Autodesk Inventor part; units mm, degrees
ref_plane "YZ Plane" through (0, 0, 0) normal (1, 0, 0) x (0, 1, 0)
ref_plane "XZ Plane" through (0, 0, 0) normal (0, 1, 0) x (-1, 0, 0)
ref_plane "XY Plane" through (0, 0, 0) normal (0, 0, 1) x (1, 0, 0)
sketch "Sketch1" plane through (0, 0, 0) normal (0, 0, 1) x (1, 0, 0)
  line L0 (0, 0) -> (235, 0)
  line L1 (235, 0) -> (235, 51)
  line L2 (235, 51) -> (0, 51)
  line L3 (0, 51) -> (0, 0)
  dimension "d0" = 235
  dimension "d1" = 51
extrude "Extrusion1" add sketch "Sketch1" along normal blind 5
sketch "Sketch2" plane through (0, 0, 5) normal (0, 0, 1) x (1, 0, 0)
  line L0 (0, 0) -> (235, 0)
  line L1 (235, 0) -> (235, 51)
  line L2 (235, 51) -> (0, 51)
  line L3 (0, 51) -> (0, 0)
  line L4 (235, 0) -> (235, 51)
  line L5 (0, 22.5) -> (235, 22.5)
  line L6 (235, 22.5) -> (235, 28.5)
  line L7 (235, 28.5) -> (0, 28.5)
  line L8 (0, 28.5) -> (0, 22.5)
  line L9 (0, 22.5) -> (235, 28.5) construction
  line L10 (235, 22.5) -> (0, 28.5) construction
  point P0 (117.5, 25.5)
  dimension "d4" = 6
extrude "Extrusion2" add sketch "Sketch2" along normal blind 3 contours L3 L7 L1 L5
sketch "Sketch3" plane through (0, 0, 5) normal (0, 0, 1) x (1, 0, 0)
  line L0 (0, 28.5) -> (235, 28.5)
  line L1 (235, 51) -> (0, 51)
  line L2 (34.5, 28.5) -> (39.5, 28.5)
  line L3 (39.5, 28.5) -> (39.5, 51)
  line L4 (39.5, 51) -> (34.5, 51)
  line L5 (34.5, 51) -> (34.5, 28.5)
  point P0 (0, 0)
  dimension "d7" = 5
sketch "Sketch5" plane through (0, 0, 5) normal (0, 0, 1) x (1, 0, 0)
  line L0 (235, 51) -> (0, 51)
  line L1 (117.5, 51) -> (117.5, 0)
  line L2 (235, 28.5) -> (0, 28.5)
  line L3 (34.5, 51) -> (39.5, 51)
  line L4 (39.5, 51) -> (39.5, 28.5)
  line L5 (39.5, 28.5) -> (34.5, 28.5)
  line L6 (34.5, 28.5) -> (34.5, 51)
  line L7 (0, 22.5) -> (235, 22.5)
  line L8 (34.5, 22.5) -> (39.5, 22.5)
  line L9 (39.5, 22.5) -> (39.5, 0)
  line L10 (39.5, 0) -> (34.5, 0)
  line L11 (34.5, 0) -> (34.5, 22.5)
  line L12 (195.5, 51) -> (195.5, 28.5)
  line L13 (200.5, 28.5) -> (200.5, 51)
  line L14 (195.5, 22.5) -> (195.5, 0)
  line L15 (195.5, 0) -> (200.5, 0)
  line L16 (200.5, 0) -> (200.5, 22.5)
  line L17 (195.5, 28.5) -> (200.5, 28.5)
  line L18 (195.5, 22.5) -> (200.5, 22.5)
  line L19 (195.5, 51) -> (200.5, 51)
  point P0 (0, 0)
  dimension "d13" = 5
extrude "Extrusion5" add sketch "Sketch3" along normal blind 3
extrude "Extrusion6" add sketch "Sketch5" along normal blind 3 contours L9 L10 L11 L7
extrude "Extrusion7" add sketch "Sketch5" along normal blind 3 contours L13 L2 L12 L0 | L7 L16 L15 L14
sketch "Sketch8" plane through (0, 0, 5) normal (0, 0, 1) x (1, 0, 0)
  circle A0 centre (29.5, 5.625) radius 1.6
  circle A1 centre (19.5, 16.875) radius 1.6
  line L0 (39.5, 0) -> (39.5, 22.5)
  line L1 (34.5, 22.5) -> (34.5, 0)
  line L2 (0, 0) -> (34.5, 0)
  dimension "d24" = 3.2
  dimension "d25" = 3.2
  dimension "d27" = 5
  dimension "d28" = 5.625
  dimension "d29" = 15
  dimension "d30" = 16.875
extrude "Extrusion9" cut sketch "Sketch8" against normal blind 10
sketch "Sketch9" plane through (0, 0, 8) normal (0, 0, 1) x (1, 0, 0)
  line L0 (0, 51) -> (0, 0)
  line L1 (0, 25.5) -> (235, 25.5)
  line L2 (235, 0) -> (235, 51)
  line L3 (117.5, 25.5) -> (117.5, -30.3106)
ref_plane "Work Plane1" through (0, 25.5, 8) normal (0, 1, 0) x (1, 0, 0)
mirror "Mirror1" about plane through (0, 25.5, 8) normal (0, 1, 0) of "Extrusion9"
ref_plane "Work Plane2" through (117.5, 25.5, 8) normal (1, 0, 0) x (0, -1, 0)
mirror "Mirror2" about plane through (117.5, 25.5, 8) normal (1, 0, 0) of "Extrusion9", "Mirror1"
sketch "Sketch11" plane through (0, 0, 5) normal (0, 0, 1) x (1, 0, 0)
  circle A0 centre (19.5, 16.875) radius 1.6
  circle A1 centre (19.5, 16.875) radius 2.1
  circle A2 centre (29.5, 5.625) radius 1.6
  circle A3 centre (29.5, 5.625) radius 2.1
  point P0 (0, 0)
  dimension "d35" = 4.2
  dimension "d36" = 4.2
extrude "Extrusion10" cut sketch "Sketch11" against normal blind 10 contours A0 | A1 | A2 | A3
mirror "Mirror3" about plane through (0, 25.5, 8) normal (0, 1, 0) of "Extrusion10"
mirror "Mirror4" about plane through (117.5, 25.5, 8) normal (1, 0, 0) of "Extrusion10", "Mirror3"
fillet "Fillet1" radius 2 4 edges at (235, 51, 2.5) (0, 51, 2.5) (0, 0, 2.5) (235, 0, 2.5)
sketch "Sketch12" plane through (0, 0, 5) normal (0, 0, 1) x (1, 0, 0)
  point P0 (0, 0)
properties part number "Impact Plate" material "ABS Plastic"
CAD build for the part. Positions are in the model's coordinates, mm. A direction names the side the tool comes from. Round coordinates to 2 decimals unless told otherwise and drop trailing zeros. Write each loop counter-clockwise with the first axis right and the second up, starting at its lowest first coordinate (ties: lowest second). Pieces come first, ordered by that corner, then holes. Notation, with made-up numbers: (58, -27.5) -> (73, -27.5) arc R24 ccw to (73, 8.5) -> close; hole circle Ø11 at (86.5, 25.25). An arc over 180 degrees is marked (long way). Answer in a Markdown table with one row per item. Add a question column.
Item 1: Drill centre lines: line 1 (Y direction, x = 215.5, z = 2.65) (3 decimals); line 2 (Y direction, x = 29.5, z = 1.95) (3 decimals); line 3 (X direction, y = 32.5, z = 1). Where is each one in solid material? Low to high. Write a range as from..to.
Item 2: Drop flat-ended pins along their axis: pin 1 Ø4 at (x, y) = (120, 13) entering from +Z; pin 2 Ø3.5 at (x, y) = (215.5, 34.125) entering from +Z; pin 3 Ø0.9 at (x, z) = (132.5, 6) entering from -Y; pin 4 Ø0.9 at (y, z) = (9, 6.5) entering from -X. Give the stop position or say it passes through.
Item 3: Mould opens along X. For faces 1 (the face through (100, 26, 8)), 2 (the face through (0, 26, 3)), 3 (the face through (217.6, 16.8, 2.5)) say: pulls with the +X half, pulls with the -X half, needs draft (parallel to the pull), parting line crosses it, or undercut.
Item 4: Saw through at A-A, the plane x = 205.5. Write the cut outline in (y, z) (3 decimals).
Item 5: Which spindle directions (+Z, -Z, +X, -X, +Y, -Y) get a long thin tool onto all of the face, cutting with end or side? Do faces 4 (the face through (218, 40, 5)), 5 (the face through (17, 40, 5)), 6 (the face through (116, 40, 5)), 7 (the face through (116, 11, 5)), 8 (the face through (218, 11, 5)). Say none if no direction does.
Findings below:
| question | item | result |
|---|---|---|
| 1 | line 1 | y = 0..14.775, 18.975..32.025, 36.225..51 |
| 1 | line 2 | y = 0..3.525, 7.725..43.275, 47.475..51 |
| 1 | line 3 | x = 0..18.17, 20.83..214.17, 216.83..235 |
| 2 | pin 1 | stops at z = 5 |
| 2 | pin 2 | passes through |
| 2 | pin 3 | stops at y = 22.5 |
| 2 | pin 4 | stops at x = 34.5 |
| 3 | face 1 | needs draft |
| 3 | face 2 | pulls with the -X half |
| 3 | face 3 | undercut |
| 4 | outline | (0, 0) -> (3.525, 0) -> (3.525, 5) -> (0, 5) -> close; (7.725, 0) -> (43.275, 0) -> (43.275, 5) -> (28.5, 5) -> (28.5, 8) -> (22.5, 8) -> (22.5, 5) -> (7.725, 5) -> close; (47.475, 0) -> (51, 0) -> (51, 5) -> (47.475, 5) -> close |
| 5 | face 4 | +Z, +X, +Y |
| 5 | face 5 | +Z, -X, +Y |
| 5 | face 6 | +Z, +Y |
| 5 | face 7 | +Z, -Y |
| 5 | face 8 | +Z, +X, -Y |
